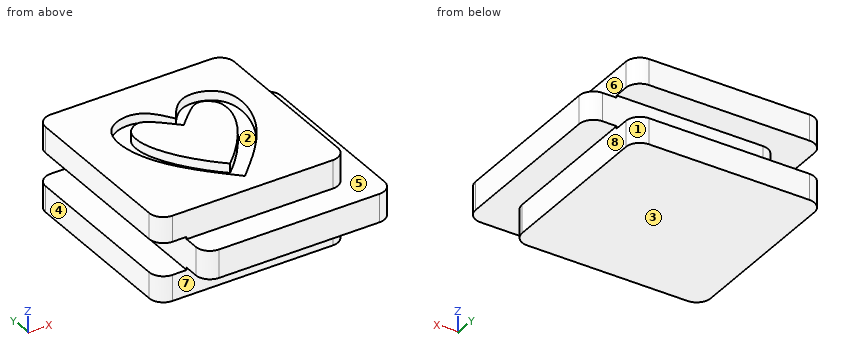
```python
from build123d import *

# Parameters (mm, degrees)
F0_W     = 14
F0_H     = 3
F0_W_2   = 3
F1_DEPTH = 20
F2_DEPTH = 3
F3_W     = 3
F3_H     = 3
F4_DEPTH = 100
F5_W     = 3
F5_H     = 3.5
F6_DEPTH = 100
F7_R     = 1.5
F9_DEPTH = 1


with BuildPart() as f1:
    # F0 (on Front) → F1 (new body)
    with BuildSketch(Plane.XZ):
        Polygon((10, 1.5), (10, 4.5), (-10, 4.5), (-10, 1.5), (-7, 1.5), (7, 1.5), align=None)
        Rectangle(F0_W, F0_H)
        with Locations((11.5, 0)):
            Rectangle(F0_W_2, F0_H)
        with Locations((8.5, 0)):
            Rectangle(F0_W_2, F0_H)
        with Locations((-8.5, 0)):
            Rectangle(F0_W_2, F0_H)
        Polygon((10, -4.5), (10, -1.5), (7, -1.5), (-7, -1.5), (-10, -1.5), (-10, -4.5), align=None)
    extrude(amount=-F1_DEPTH)

    # F0 (on Front) → F2 (join)
    with BuildSketch(Plane.XZ):
        with Locations((-8.5, 0)):
            Rectangle(F0_W_2, F0_H)
        Rectangle(F0_W, F0_H)
        with Locations((8.5, 0)):
            Rectangle(F0_W_2, F0_H)
        with Locations((11.5, 0)):
            Rectangle(F0_W_2, F0_H)
    extrude(amount=F2_DEPTH)

    # F3 (on face) → F4 (cut)
    with BuildSketch(Plane.YZ.offset(13)):
        Polygon((23, -1.75), (23, 1.75), (17, 1.75), (17, 1.5), (20, 1.5), (20, -1.5), (17, -1.5), (17, -1.75), align=None)
        with Locations((18.5, 0)):
            Rectangle(F3_W, F3_H)
    extrude(amount=-F4_DEPTH, mode=Mode.SUBTRACT)

    # F5 (on face) → F6 (cut)
    with BuildSketch(Plane(origin=(0, 17, 0), x_dir=(-1, 0, 0), z_dir=(0, 1, 0))):
        with Locations((11.5, 0)):
            Rectangle(F5_W, F5_H)
        with Locations((8.5, 0)):
            Rectangle(F5_W, F5_H)
    extrude(amount=-F6_DEPTH, mode=Mode.SUBTRACT)

    # F7
    f7_edges = [f1.edges().sort_by_distance(p)[0] for p in [
        (-7, -3, 0),
        (13, -3, 0),
        (10, 0, 3),
        (10, 0, -3),
        (-10, 0, -3.125),
        (-10, 0, 3.125),
        (-7, 17, 0),
        (-10, 20, 3.125),
        (-10, 20, -3.125),
        (13, 17, 0),
        (10, 20, 3.125),
        (10, 20, -3.125),
    ]]
    fillet(f7_edges, radius=F7_R)

    # F8 (on face) → F9 (cut)
    with BuildSketch(Plane.XY.offset(4.5)):
        with BuildLine():
            Line((0.5079321563, 12.6308239996), (0.5079321563, 13.3923562244))
            add(Edge.make_bspline(
                [(0.5079321563, 13.3923562244), (-0.2042453086, 14.4841945601), (-1.6194856249, 16.653897794), (-6.4925619551, 15.4160387293), (-5.8372524097, 8.372899764), (-1.7703990856, 4.3107311976), (0.5079321563, 2.0350255072)],
                knots=[0, 0, 0, 0, 0.2063930363, 0.4101447224, 0.6695517086, 1, 1, 1, 1], degree=3))
            Line((0.5079321563, 2.0350255072), (0.5079321563, 3.2167136669))
            add(Edge.make_bspline(
                [(0.5079321563, 12.6308239996), (-0.2166217589, 13.5477579815), (-1.4496563968, 15.1081819987), (-3.2014964515, 15.467028439), (-5.0022320005, 14.3189482089), (-5.3079861121, 11.6387311218), (-3.4341416808, 7.1131911239), (-0.8432740412, 4.5522916121), (0.5079321563, 3.2167136669)],
                knots=[0, 0, 0, 0, 0.169604223, 0.2886298612, 0.4171601384, 0.5655007654, 0.7733969919, 1, 1, 1, 1], degree=3))
        make_face()
        with BuildLine():
            add(Edge.make_bspline(
                [(0.5079321563, 13.3923562244), (1.2201096213, 14.4841945601), (2.6353499375, 16.653897794), (7.5084262677, 15.4160387293), (6.8531167223, 8.372899764), (2.7862633983, 4.3107311976), (0.5079321563, 2.0350255072)],
                knots=[0, 0, 0, 0, 0.2063930363, 0.4101447224, 0.6695517086, 1, 1, 1, 1], degree=3))
            Line((0.5079321563, 13.3923562244), (0.5079321563, 12.6308239996))
            add(Edge.make_bspline(
                [(0.5079321563, 12.6308239996), (1.2324860716, 13.5477579815), (2.4655207094, 15.1081819987), (4.2173607642, 15.467028439), (6.0180963131, 14.3189482089), (6.3238504248, 11.6387311218), (4.4500059934, 7.1131911239), (1.8591383538, 4.5522916121), (0.5079321563, 3.2167136669)],
                knots=[0, 0, 0, 0, 0.169604223, 0.2886298612, 0.4171601384, 0.5655007654, 0.7733969919, 1, 1, 1, 1], degree=3))
            Line((0.5079321563, 3.2167136669), (0.5079321563, 2.0350255072))
        make_face()
        with BuildLine():
            add(Edge.make_bspline(
                [(0.5079321563, 12.6308239996), (1.2324860716, 13.5477579815), (2.4655207094, 15.1081819987), (4.2173607642, 15.467028439), (6.0180963131, 14.3189482089), (6.3238504248, 11.6387311218), (4.4500059934, 7.1131911239), (1.8591383538, 4.5522916121), (0.5079321563, 3.2167136669)],
                knots=[0, 0, 0, 0, 0.169604223, 0.2886298612, 0.4171601384, 0.5655007654, 0.7733969919, 1, 1, 1, 1], degree=3))
            Line((0.5079321563, 12.6308239996), (0.5079321563, 12.1036916971))
            add(Edge.make_bspline(
                [(0.5079321563, 12.1036916971), (0.9845350772, 12.5783972914), (1.9182678659, 13.5084136695), (3.5364426534, 14.9021637489), (4.7681552632, 14.1418940477), (5.3308142058, 13.4027101407), (5.4419389667, 11.3924890124), (3.9669526492, 8.2792374371), (1.784815358, 5.6918019484), (0.880360239, 4.8502334126), (0.5079321563, 4.5036990196)],
                knots=[0, 0, 0, 0, 0.1285135055, 0.2517762593, 0.348617425, 0.4320442691, 0.5523455091, 0.7197270075, 0.8845921433, 1, 1, 1, 1], degree=3))
            Line((0.5079321563, 4.5036990196), (0.5079321563, 3.2167136669))
        make_face()
        with BuildLine():
            Line((0.5079321563, 12.1036916971), (0.5079321563, 12.6308239996))
            add(Edge.make_bspline(
                [(0.5079321563, 12.6308239996), (-0.2166217589, 13.5477579815), (-1.4496563968, 15.1081819987), (-3.2014964515, 15.467028439), (-5.0022320005, 14.3189482089), (-5.3079861121, 11.6387311218), (-3.4341416808, 7.1131911239), (-0.8432740412, 4.5522916121), (0.5079321563, 3.2167136669)],
                knots=[0, 0, 0, 0, 0.169604223, 0.2886298612, 0.4171601384, 0.5655007654, 0.7733969919, 1, 1, 1, 1], degree=3))
            Line((0.5079321563, 3.2167136669), (0.5079321563, 4.5036990196))
            add(Edge.make_bspline(
                [(0.5079321563, 12.1036916971), (0.0313292355, 12.5783972914), (-0.9024035532, 13.5084136695), (-2.5205783407, 14.9021637489), (-3.7522909505, 14.1418940477), (-4.3149498931, 13.4027101407), (-4.426074654, 11.3924890124), (-2.9510883366, 8.2792374371), (-0.7689510454, 5.6918019484), (0.1355040736, 4.8502334126), (0.5079321563, 4.5036990196)],
                knots=[0, 0, 0, 0, 0.1285135055, 0.2517762593, 0.348617425, 0.4320442691, 0.5523455091, 0.7197270075, 0.8845921433, 1, 1, 1, 1], degree=3))
        make_face()
    extrude(amount=-F9_DEPTH, mode=Mode.SUBTRACT)


solid = f1.part
```
Model file for the job. Use its own axes, mm. Face numbers are marked on the shaded views. A direction names the side the tool comes from. Coordinates: 2 decimals unless noted, no trailing zeros. Loops run counter-clockwise (first coordinate to the right, second up) from the corner with the lowest first, then second, coordinate; pieces in that order, holes last. Notation, with made-up numbers: (10.5, 81) - (17.5, 81) arc R28 cw to (17.5, 103) - close; hole circle Ø2 at (64, -1). An arc over 180 degrees is marked (long way). Answer as a JSON object with one key per item and string values. Group by question number.
(1) Two-plate mould, pull along X, no slides. Class the marked faces 1, 2, 3 and 4: released by +X, released by -X, zero draft, split by the parting line, or undercut.
(2) Cut at A-A (z = -2.25). Give the cut face in (x, y), then the cut area to 3 significant figures.
(3) Cut at B-B (y = -1). Give the cut face in (x, z).
(4) Probe line 1 along Z through (x, y) = (-3.75, 17.5); line 2 along Y through (x, z) = (3, 4); line 3 along X through (y, z) = (5, -0.25). List the from-to ranges inside material, lowest first.
(5) Tool access for the marked faces 5, 6, 7 and 8: list every direction of +Z, -Z, +X, -X, +Y, -Y with a clear straight run to the whole face (end or side of a thin tool).
(6) Flat gauge pins, fed straight in: pin 1 (1.8 mm diameter, centred on y = 6, z = -0.5, fed in from -X); pin 2 (1.5 mm diameter, centred on x = 3, z = 3, fed in from -Y); pin 3 (0.9 mm diameter, centred on y = 8.5, z = 3.5, fed in from +X). Where does each tip first touch, or does it go through?
Geometry says:
{
 "1": {"face 1": "released by +X", "face 2": "undercut", "face 3": "zero draft", "face 4": "released by -X"},
 "2": {"outline": "(-10, 1.5) arc R1.5 ccw to (-8.5, 0) - (8.5, 0) arc R1.5 ccw to (10, 1.5) - (10, 18.5) arc R1.5 ccw to (8.5, 20) - (-8.5, 20) arc R1.5 ccw to (-10, 18.5) - close", "area": "398 mm^2"},
 "3": {"outline": "(-7, -1.5) - (13, -1.5) - (13, 1.5) - (-7, 1.5) - close"},
 "4": {"line 1": "z = -4.5 to -1.75, 1.75 to 4.5", "line 2": "y = 0 to 4.6, 7.19 to 14.34, 15.91 to 20", "line 3": "x = -7 to 13"},
 "5": {"face 5": "+Z, +X, -Y", "face 6": "+Z, +X, +Y, -Y", "face 7": "-Z, +X, -X, -Y", "face 8": "-Z, +X, +Y, -Y"},
 "6": {"pin 1": "stops at x = -7", "pin 2": "stops at y = 0", "pin 3": "stops at x = 10"}
}
